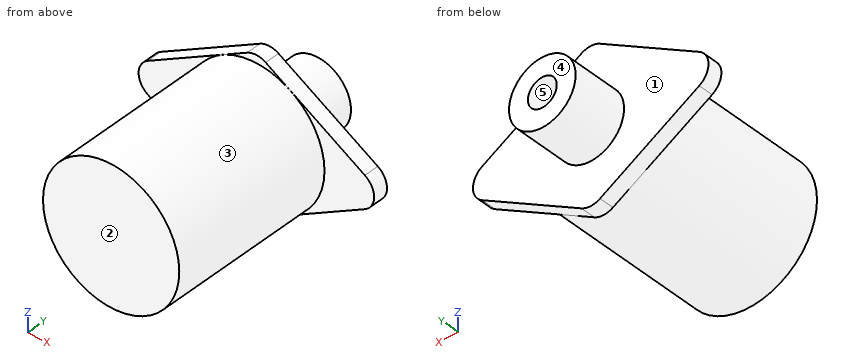
```python
from build123d import *

# Parameters (mm, degrees)
SKETCH1_R           = 18.4
BOSS_EXTRUDE1_DEPTH = 45
BOSS_EXTRUDE2_DEPTH = 4
FILLET1_R           = 5
SKETCH3_R           = 9
BOSS_EXTRUDE3_DEPTH = 15
SKETCH4_R           = 3.9
CUT_EXTRUDE1_DEPTH  = 10


with BuildPart() as part:
    # Sketch1 → Boss-Extrude1 (new body)
    with BuildSketch(Plane(origin=(0, 0, 0), x_dir=(1, 0, 0), z_dir=(0, 1, 0))):
        Circle(SKETCH1_R)
    extrude(amount=BOSS_EXTRUDE1_DEPTH)

    # Sketch2 → Boss-Extrude2 (add)
    with BuildSketch(Plane(origin=(0, 45, 0), x_dir=(1, 0, 0), z_dir=(0, 1, 0))):
        Polygon((0, 21.25), (-36.806079661, 0), (0, -21.25), (36.806079661, 0), align=None)
    extrude(amount=BOSS_EXTRUDE2_DEPTH)

    # Fillet1
    fillet1_edges = [part.edges().sort_by_distance(p)[0] for p in [
        (36.806079661, 47, 0),
        (0, 47, -21.25),
        (-36.806079661, 47, 0),
        (0, 47, 21.25),
    ]]
    fillet(fillet1_edges, radius=FILLET1_R)

    # Sketch3 → Boss-Extrude3 (add)
    with BuildSketch(Plane(origin=(0, 49, 0), x_dir=(1, 0, 0), z_dir=(0, 1, 0))):
        Circle(SKETCH3_R)
    extrude(amount=BOSS_EXTRUDE3_DEPTH)

    # Sketch4 → Cut-Extrude1 (cut)
    with BuildSketch(Plane(origin=(0, 64, 0), x_dir=(1, 0, 0), z_dir=(0, 1, 0))):
        Circle(SKETCH4_R)
    extrude(amount=-CUT_EXTRUDE1_DEPTH, mode=Mode.SUBTRACT)


solid = part.part
```
CAD build for the part. Positions are in the model's coordinates, mm. Face numbers are marked on the shaded views. A direction names the side the tool comes from. Give positions to 0.01 mm unless a question says otherwise; leave off trailing zeros. Order: outer loops, then holes, each group sorted by start corner. A loop starts at its lowest first (then second) coordinate and runs counter-clockwise, first axis right, second up.
(1) Saw through at A-A, the plane x = 0. Give the cut face in (y, z), then the cut area to 3 significant figures.
(2) Saw through at D-D, the plane z = 17.5. Give the cut face in (x, y), then the cut area to 3 significant figures.
(3) Saw through at C-C, the plane z = 0. Give the cut face in (x, y), then the cut area to 3 significant figures.
(4) Tool access for the marked faces 1 and 2: list every direction of +Z, -Z, +X, -X, +Y, -Y with a clear straight run to the whole face (end or side of a thin tool).
(5) Mould opens along X. For the marked faces 3, 4 and 5 say: released by +X, released by -X, zero draft, split by the parting line, or undercut.
(6) Drill centre lines: L1, parallel to Z at x = 0, y = 59.75; L2, parallel to Y at x = -17, z = -3. Where is each one in solid material? Low to high.
(7) Saw through at B-B, the plane y = 46. Give the cut face in (x, z).
(8) Flat gauge pins, fed straight in: pin 1 (7 mm diameter, centred on x = 0, z = 0, fed in from +Y); pin 2 (5 mm diameter, centred on y = 34, z = -6.5, fed in from -X); pin 3 (4 mm diameter, centred on x = 13.5, z = -1.5, fed in from -Y); pin 4 (10 mm diameter, centred on x = -6.5, y = 37, fed in from +Z). Where does each tip first touch, or does it go through?
Results found:
1. outline: (0, -18.4) - (45, -18.4) - (45, -20.48) - (49, -20.48) - (49, -9) - (64, -9) - (64, -3.9) - (54, -3.9) - (54, 3.9) - (64, 3.9) - (64, 9) - (49, 9) - (49, 20.48) - (45, 20.48) - (45, 18.4) - (0, 18.4) - close
1. area: 2,010 mm2
2. outline: (-6.5, 45) - (-5.68, 45) - (-5.68, 0) - (5.68, 0) - (5.68, 45) - (6.5, 45) - (6.5, 49) - (-6.5, 49) - close
2. area: 564 mm2
3. outline: (-31.81, 45) - (-18.4, 45) - (-18.4, 0) - (18.4, 0) - (18.4, 45) - (31.81, 45) - (31.81, 49) - (9, 49) - (9, 64) - (3.9, 64) - (3.9, 54) - (-3.9, 54) - (-3.9, 64) - (-9, 64) - (-9, 49) - (-31.81, 49) - close
3. area: 2,100 mm2
4. face 1: +Y
4. face 2: +Z, -Z, +X, -X, -Y
5. face 3: split by the parting line
5. face 4: zero draft
5. face 5: undercut
6. L1: z = -9 to -3.9, 3.9 to 9
6. L2: y = 0 to 49
7. outline: (-29.31, -4.33) - (-2.5, -19.81) arc R5 ccw to (2.5, -19.81) - (29.31, -4.33) arc R5 ccw to (29.31, 4.33) - (2.5, 19.81) arc R5 ccw to (-2.5, 19.81) - (-29.31, 4.33) arc R5 ccw to start
8. pin 1: stops at y = 54
8. pin 2: stops at x = -17.96
8. pin 3: stops at y = 0
8. pin 4: stops at z = 18.34
